```python
from build123d import *

# Parameters (mm, degrees)
F0_R     = 12.5
F1_DEPTH = 5
F3_DEPTH = 5
F4_R     = 1.27
F5_COUNT = 12
F6_R     = 7.62
F7_DEPTH = 25.4


with BuildPart() as f1:
    # F0 (on Front) → F1 (new body)
    with BuildSketch(Plane.XZ):
        Circle(F0_R)
    extrude(amount=F1_DEPTH)

    # F2 (on face) → F3 (join, through all)
    with BuildSketch(Plane.XZ.offset(5)):
        with BuildLine():
            ThreePointArc((-2.54, 12.2392156611), (0, 12.5), (2.54, 12.2392156611))
            ThreePointArc((2.54, 12.2392156611), (2.3217431159, 15.5720988713), (0.889, 18.5892156611))
            Line((0.889, 18.5892156611), (-0.889, 18.5892156611))
            ThreePointArc((-0.889, 18.5892156611), (-2.3217431159, 15.5720988713), (-2.54, 12.2392156611))
        make_face()
    extrude(amount=-F3_DEPTH)

    # F4
    f4_edges = [f1.edges().sort_by_distance(p)[0] for p in [
        (-0.889, -2.5, 18.589216),
        (0.889, -2.5, 18.589216),
    ]]
    fillet(f4_edges, radius=F4_R)

    # F5: F1 ×12 about axis
    f5_axis = Axis((0, 0, 0), (0, 1, 0))


with BuildPart() as f1_1:
    add(f1.part)
    for i in range(1, F5_COUNT):
        add(f1.part.rotate(f5_axis, i * 360 / F5_COUNT))

    # F6 (on face) → F7 (cut)
    with BuildSketch(Plane.XZ.offset(5)):
        Circle(F6_R)
    extrude(amount=-F7_DEPTH, mode=Mode.SUBTRACT)


solid = f1_1.part
```
Here's how the part is built. I have some questions about the finished solid (model axes, mm). A direction names the side the tool comes from. Coordinates: 2 decimals unless noted, no trailing zeros. Order: outer loops, then holes, each group sorted by start corner. A loop starts at its lowest first (then second) coordinate and runs counter-clockwise, first axis right, second up.
Item 1: Which directions (+Z, -Z, +X, -X, +Y, -Y) give clear straight access to the entire face, cutting with the end or side of a thin tool? Please do faces 1 (the face through (-9.93, -2.46, 15.55)), 2 (the face through (-2.397, -2.535, 15.258)), 3 (the face through (-14.35, -2.535, -5.496)).
Response values:
face 1: +Z, -X, +Y, -Y
face 2: +Y, -Y
face 3: -X, +Y, -Y
Item 2: I'm going to push flat-ended pins straight in: pin 1 Ø2 at (y, z) = (-2.5, -2.5) entering from +X; pin 2 Ø1.5 at (x, y) = (-2.5, -0.5) entering from +Z. Where does each tip first touch, or does it pass through?
Response values:
pin 1: stops at x = 17.63
pin 2: stops at z = 17.15
Item 3: If we section it at C-C, the plane z = 13.5: List the corners of the cut face in (x, y) for me.
Response values:
outline: (-10.04, -5) - (-4.82, -5) - (-4.82, 0) - (-10.04, 0) - close; (-2.61, -5) - (2.61, -5) - (2.61, 0) - (-2.61, 0) - close; (4.82, -5) - (10.04, -5) - (10.04, 0) - (4.82, 0) - close
Item 4: If we section it at A-A, the plane z = -7: List the corners of the cut face in (x, y) for me, then the cut area to 3 significant figures.
Response values:
outline: (-15.68, -5) - (-3.01, -5) - (-3.01, 0) - (-15.68, 0) - close; (3.01, -5) - (15.68, -5) - (15.68, 0) - (3.01, 0) - close
area: 127 mm2
Item 5: If we section it at B-B, the plane x = -7: List the corners of the cut face in (y, z) for me, then the cut area to 3 significant figures.
Response values:
outline: (-5, -15.68) - (0, -15.68) - (0, -3.01) - (-5, -3.01) - close; (-5, 3.01) - (0, 3.01) - (0, 15.68) - (-5, 15.68) - close
area: 127 mm2
Item 6: I need wall thicknesses on probe 1 along Z at (x, y) = (0, -3.55); probe 2 along X at (y, z) = (-0.15, -15); probe 3 along Z at (x, y) = (16, -4.3). Which ranges of each line are inside material? Lowest first, please.
Response values:
probe 1: z = -18.59 to -7.62, 7.62 to 18.59
probe 2: x = -10.11 to -6.14, -2.45 to 2.45, 6.14 to 10.11
probe 3: z = -9.47 to -7.48, -2.2 to 2.2, 7.48 to 9.47
Item 7: Thinking about a two-plate mould opening in X: for faces 4 (the face through (18.423, -2.465, -0.841)), 5 (the face through (-16.375, -2.465, -8.483)), 6 (the face through (2.397, -2.535, -15.258)), which applies, pulls with the +X half, pulls with the -X half, needs draft (parallel to the pull), parting line crosses it, or undercut?
Response values:
face 4: pulls with the +X half
face 5: pulls with the -X half
face 6: undercut
